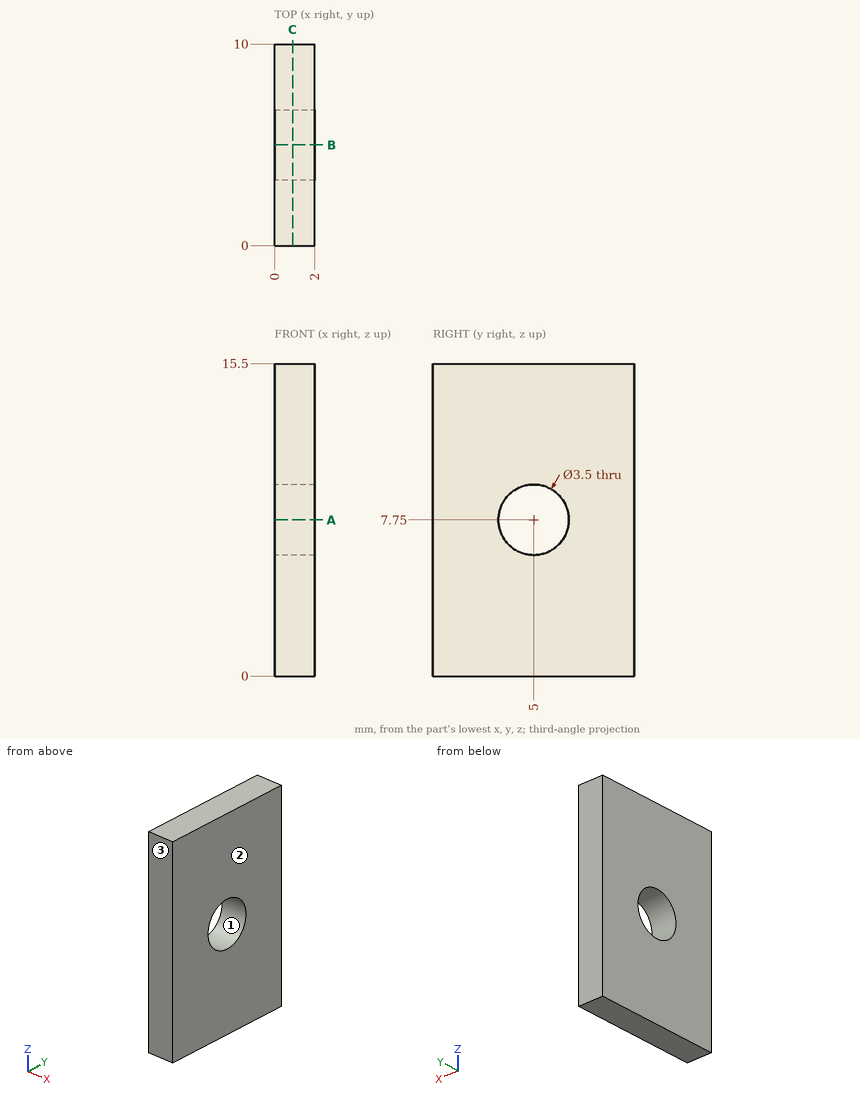
Check sheet for the drawn part. Datum: minimum x, y, z corner. Units: mm. Round coordinates to 2 decimals unless told otherwise and drop trailing zeros. Order: outer loops, then holes, each group sorted by start corner. A loop starts at its lowest first (then second) coordinate and runs counter-clockwise, first axis right, second up. Notation, with made-up numbers: (54.5, 48.25) -> (97.5, 48.25) arc R26 cw to (97.5, 72.25) -> close; hole circle Ø11 at (-19.5, 53). An arc over 180 degrees is marked (long way). Return JSON: item names as keys, results as strings. Group by question number.
Q1. Section check C-C, the plane x = 0.9. Record the boundary of the cut face in (y, z), plus the area to 3 significant figures.
Q2. Section check B-B, the plane y = 5. Record the boundary of the cut face in (x, z).
Q3. Material ranges on probe 1 along Z at (x, y) = (1.1, 5); probe 2 along Y at (x, z) = (1.45, 7.75); probe 3 along Y at (x, z) = (1.75, 9), recorded low to high. Write a range as from..to.
Q4. Release check for a two-part mould opening along Y. For the marked faces 1, 2 and 3 record: released by +Y, released by -Y, zero draft, split by the parting line, or undercut.
Q5. Section check A-A, the plane z = 7.75. Record the boundary of the cut face in (x, y), plus the area to 3 significant figures.
Q6. Gauge pin test, flat end, axial feed: pin 1 (3 mm diameter, centred on y = 5, z = 7.75, fed in from +X). Record the tip position at first contact, or that the pin passes through.
Numbers:
{
 "1": {"outline": "(0, 0) -> (10, 0) -> (10, 15.5) -> (0, 15.5) -> close; hole circle Ø3.5 at (5, 7.75)", "area": "145 mm^2"},
 "2": {"outline": "(0, 0) -> (2, 0) -> (2, 6) -> (0, 6) -> close; (0, 9.5) -> (2, 9.5) -> (2, 15.5) -> (0, 15.5) -> close"},
 "3": {"probe 1": "0..6, 9.5..15.5", "probe 2": "0..3.25, 6.75..10", "probe 3": "0..3.78, 6.22..10"},
 "4": {"face 1": "undercut", "face 2": "zero draft", "face 3": "released by -Y"},
 "5": {"outline": "(0, 0) -> (2, 0) -> (2, 3.25) -> (0, 3.25) -> close; (0, 6.75) -> (2, 6.75) -> (2, 10) -> (0, 10) -> close", "area": "13.0 mm^2"},
 "6": {"pin 1": "through"}
}
